Answer from the drawing. Dimensions are ordinates in mm from the lowest x, y and z of the part. A direction names the side the tool comes from. Give positions to 0.01 mm unless a question says otherwise; leave off trailing zeros. Loops run counter-clockwise (first coordinate to the right, second up) from the corner with the lowest first, then second, coordinate; pieces in that order, holes last. Notation, with made-up numbers: M -28,71 L -9,71 A27 cw -9,92 Z; hole C 19,76.25 d7. An arc over 180 degrees is marked long. Use a Markdown table: item, result.
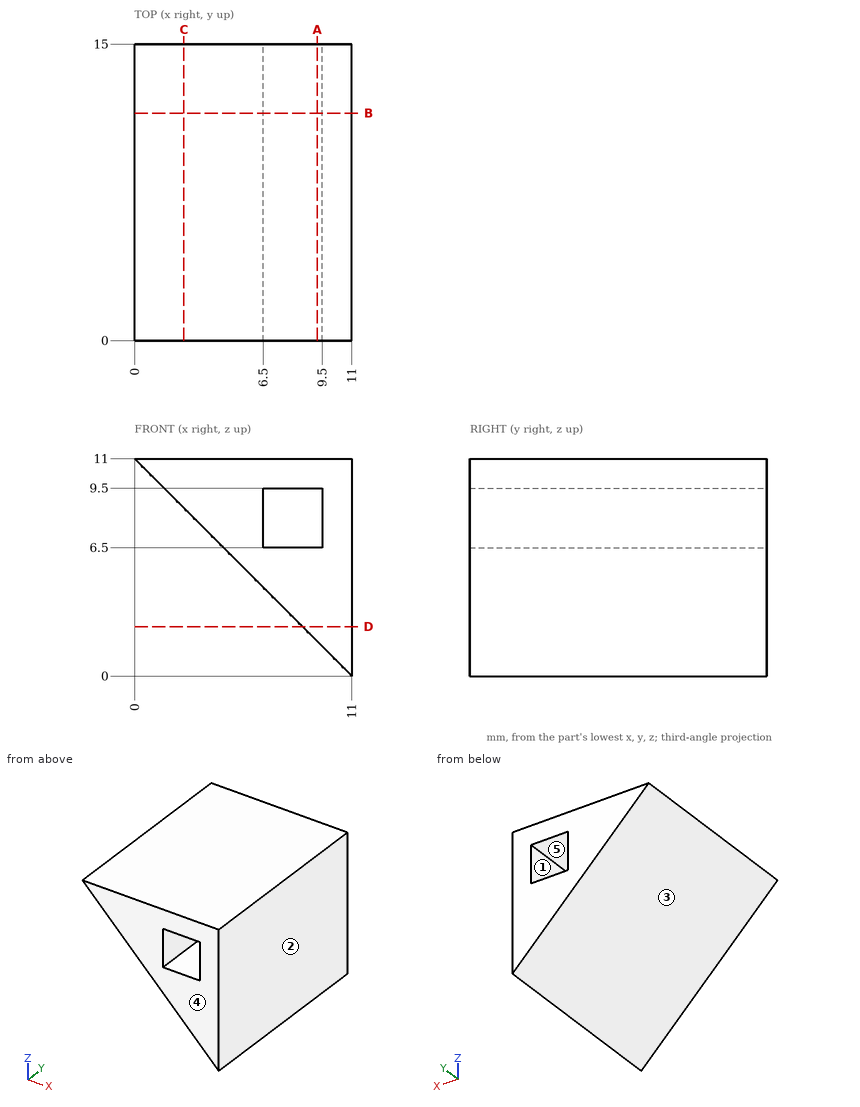
(1) A cutting plane is placed at A-A (x = 9.25). Write down the section's boundary in (y, z), and give its area (4 significant figures).
Entries:
| item | result |
|---|---|
| outline | M 0,1.75 L 15,1.75 L 15,6.5 L 0,6.5 Z; M 0,9.5 L 15,9.5 L 15,11 L 0,11 Z |
| area | 93.75 mm² |
(2) Consider probe 1 along Z at (x, y) = (1.5, 13.5); probe 2 along Z at (x, y) = (9.25, 11); probe 3 along Z at (x, y) = (8, 4.25). Determine where each line is inside the solid, lowest interval first. Write a range as [from, to].
Entries:
| item | result |
|---|---|
| probe 1 | z = [9.5, 11] |
| probe 2 | z = [1.75, 6.5], [9.5, 11] |
| probe 3 | z = [3, 6.5], [9.5, 11] |
(3) Given P1, Ø3.5, axis at y = 4, z = 8, coming from the -X side; P2, Ø2.5, axis at x = 8, y = 4, coming from the -Z side; P3, Ø3, axis at x = 4, y = 8, coming from the -Z side; P4, Ø4, axis at y = 7.5, z = 9.5, coming from the -X side, each flat-ended and moving along its own axis, determine where each tip first touches the part or whether it passes through.
Entries:
| item | result |
|---|---|
| P1 | stops at x = 1.25 |
| P2 | stops at z = 1.75 |
| P3 | stops at z = 5.5 |
| P4 | stops at x = 0 |
(4) A cutting plane is placed at B-B (y = 11.5). Write down the section's boundary in (x, z), and give its area (3 significant figures).
Entries:
| item | result |
|---|---|
| outline | M 0,11 L 11,0 L 11,11 Z; hole M 6.5,6.5 L 9.5,6.5 L 9.5,9.5 L 6.5,9.5 Z |
| area | 51.5 mm² |
(5) The mould has two halves that part along Z. Classify the marked faces 3, 4 and 5: released by +Z, released by -Z, zero draft, split by the parting line, or undercut.
Entries:
| item | result |
|---|---|
| face 3 | released by -Z |
| face 4 | zero draft |
| face 5 | undercut |
(6) Which of the six approach directions +Z, -Z, +X, -X, +Y, -Y give full straight-line access (tool end or side, diameter ignored) to the marked faces 1 and 2?
Entries:
| item | result |
|---|---|
| face 1 | +Y, -Y |
| face 2 | +Z, -Z, +X, +Y, -Y |
(7) A cutting plane is placed at D-D (z = 2.5). Write down the section's boundary in (x, y), and give its area (3 significant figures).
Entries:
| item | result |
|---|---|
| outline | M 8.5,0 L 11,0 L 11,15 L 8.5,15 Z |
| area | 37.5 mm² |
(8) A cutting plane is placed at C-C (x = 2.5). Write down the section's boundary in (y, z), and give its area (3 significant figures).
Entries:
| item | result |
|---|---|
| outline | M 0,8.5 L 15,8.5 L 15,11 L 0,11 Z |
| area | 37.5 mm² |
